Source: CAD feature listing. Evaluate the final solid. Frame: model axes, mm. Face numbers are marked on the shaded views. A direction names the side the tool comes from. Give positions to 0.01 mm unless a question says otherwise; leave off trailing zeros. Order: outer loops, then holes, each group sorted by start corner. A loop starts at its lowest first (then second) coordinate and runs counter-clockwise, first axis right, second up.
1) Section C-C, the plane z = 0.75. Return loops of the section in (x, y), plus the area to 3 significant figures.
2) Section B-B, the plane x = -43.5. Return loops of the section in (y, z), plus the area to 3 significant figures.
3) Draft query along X for the marked faces 3, 4 and 5. Return one class per face: released by +X, released by -X, zero draft, split by the parting line, or undercut.
4) Section A-A, the plane y = -9.5. Return loops of the section in (x, z), plus the area to 3 significant figures.
5) Access query for the marked faces 1 and 2. Directions: +Z, -Z, +X, -X, +Y, -Y. A direction counts if a zero-diameter tool reaches every point of the face in a straight line with its end or side. Return the directions, or none.
6) Material intervals for line 1 (X direction, y = -20, z = -0.25); line 2 (Z direction, x = 30.5, y = -9); line 3 (Y direction, x = -54, z = 5), sorted ascending.
7) First-contact query: P1, Ø10, axis at x = -33, z = 8.5, coming from the -Y side; P2, Ø6, axis at x = -5, y = -54, coming from the +Z side; P3, Ø6, axis at x = 7.5, y = -21, coming from the +Z side. Flat tips, straight axial feed; report the tip coordinate or a pass-through.
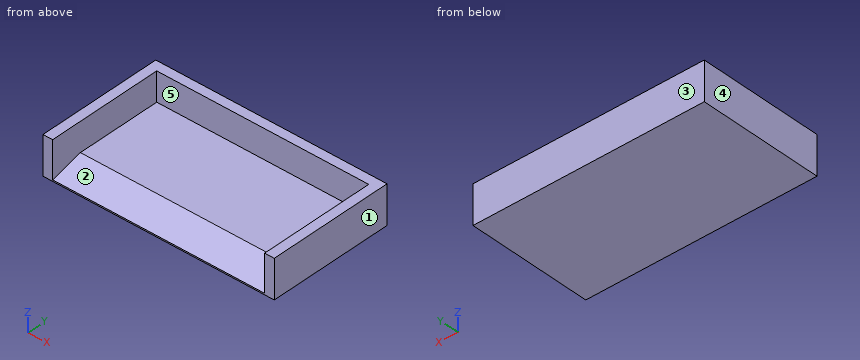
```python
from build123d import *

# Parameters (mm, degrees)
F1_DEPTH = 76.2
F2_SIZE2 = 5.444728
F2_SIZE  = 20.32
F3_W     = 152.4
F3_H     = 25.4
F4_DEPTH = 6.35


with BuildPart() as f1:
    # F0 (on Front) → F1 (new body)
    with BuildSketch(Plane.XZ):
        Polygon((69.85, -12.7), (76.2, -12.7), (76.2, 12.7), (69.85, 12.7), (69.85, -6.35), (-69.85, -6.35), (-69.85, 12.7), (-76.2, 12.7), (-76.2, -6.35), (-76.2, -12.7), align=None)
    extrude(amount=F1_DEPTH)

    # F2
    f2_edges = [f1.edges().sort_by_distance(p)[0] for p in [
        (0, -76.2, -6.35),
    ]]
    chamfer(f2_edges, length=F2_SIZE, length2=F2_SIZE2)

    # F3 (on Front) → F4 (join)
    with BuildSketch(Plane.XZ):
        Rectangle(F3_W, F3_H)
    extrude(amount=-F4_DEPTH)


solid = f1.part
```
From the geometry:
1. outline: (-76.2, -76.2) - (-69.85, -76.2) - (-69.85, 0) - (69.85, 0) - (69.85, -76.2) - (76.2, -76.2) - (76.2, 6.35) - (-76.2, 6.35) - close
1. area: 1,940 mm2
2. outline: (-76.2, -12.7) - (6.35, -12.7) - (6.35, 12.7) - (0, 12.7) - (0, -6.35) - (-55.88, -6.35) - (-76.2, -11.79) - close
2. area: 590 mm2
3. face 3: zero draft
3. face 4: released by -X
3. face 5: undercut
4. outline: (-76.2, -12.7) - (76.2, -12.7) - (76.2, 12.7) - (69.85, 12.7) - (69.85, -6.35) - (-69.85, -6.35) - (-69.85, 12.7) - (-76.2, 12.7) - close
4. area: 1,210 mm2
5. face 1: +Z, -Z, +X, +Y, -Y
5. face 2: +Z, -Y
6. line 1: x = -76.2 to -69.85, 69.85 to 76.2
6. line 2: z = -12.7 to -6.35
6. line 3: y = 0 to 6.35
7. P1: stops at y = 0
7. P2: stops at z = -6.35
7. P3: stops at z = -6.35
